The model under review builds one solid part; all positions refer to its coordinate system, in mm. Face numbers are marked on the shaded views. Round coordinates to 2 decimals unless told otherwise and drop trailing zeros. Write each loop counter-clockwise with the first axis right and the second up, starting at its lowest first coordinate (ties: lowest second). Pieces come first, ordered by that corner, then holes. Notation, with made-up numbers: M 85,61 L 126,61 A17 cw 126,91 Z; hole C -19.75,-6 d7. An arc over 180 degrees is marked long. One line per item, written item: value. Start each with the question number.
1) For P1, Ø3, axis at y = 4, z = 5, coming from the +X side; P2, Ø10, axis at x = -10, y = -1, coming from the +Z side; P3, Ø1, axis at y = 5.5, z = 5.5, coming from the +X side, all flat-tipped, find the tip position at first contact; note any pin that passes through.
2) Mouldability with a two-part tool opening along Y and no side actions: class the marked faces 1, 2, 3 and 4 as +Y half, -Y half, draft (parallel to the pull), parting line (faces both ways), or undercut.
3) Wall thickness on probe 1 along Y at (x, z) = (-14.5, 4.75); probe 2 along X at (y, z) = (-3.25, 1.75); probe 3 along X at (y, z) = (5, 3): over which ranges is each line inside the solid? List them lowest first.
4) Take a section at D-D, the plane x = 19. Write out the cut boundary in (y, z), and give its area (3 significant figures).
5) Take a section at B-B, the plane x = 9.5. Write out the cut boundary in (y, z).
6) Take a section at A-A, the plane y = 0. Write out the cut boundary in (x, z), and give its area (3 significant figures).
7) Take a section at C-C, the plane z = 3. Write out the cut boundary in (x, y), and give its area (3 significant figures).
from build123d import *

# Parameters (mm, degrees)
EXTRUDE_1_DEPTH = 7
M16X1_51_D      = 14.5


with BuildPart() as part:
    # Эскиз1 → Бобышка-Вытянуть1 (new body)
    with BuildSketch(Plane.XY):
        with BuildLine():
            Line((14.5, 9), (-14.5, 9))
            ThreePointArc((-14.5, 9), (-23.5, 0), (-14.5, -9))
            Line((-14.5, -9), (14.5, -9))
            ThreePointArc((14.5, -9), (23.5, 0), (14.5, 9))
        make_face()
    extrude(amount=EXTRUDE_1_DEPTH)

    # Отверстие обработанное метчиком M16x1.51 (through all)
    with Locations(Plane(origin=(0, 0, 0), x_dir=(-1, 0, 0), z_dir=(0, 0, -1))):
        with Locations((14.5, 0)):
            m16x1_51 = Hole(M16X1_51_D / 2)

    # Зеркальное отражение1: Отверстие обработанное метчиком M16x1.51 across plane
    add(m16x1_51.mirror(Plane(origin=(0, 0, 0), x_dir=(0, 0, 1), z_dir=(1, 0, 0))), mode=Mode.SUBTRACT)


solid = part.part
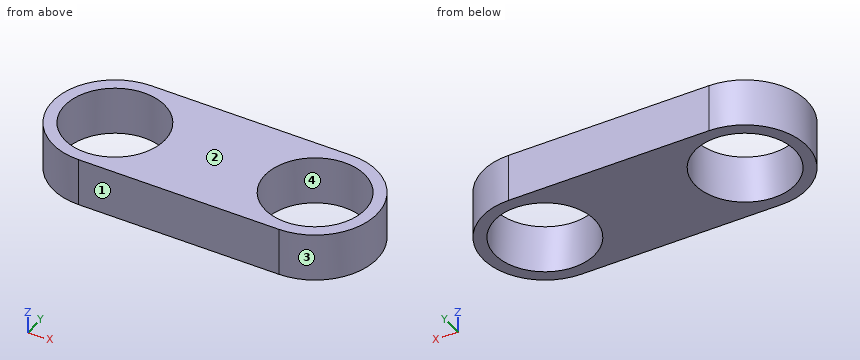
Checked values:
1. P1: stops at x = 23.15
1. P2: stops at z = 7
1. P3: stops at x = 21.98
2. face 1: -Y half
2. face 2: draft
2. face 3: parting line
2. face 4: undercut
3. probe 1: y = -9 to -7.25, 7.25 to 9
3. probe 2: x = -22.89 to -20.98, -8.02 to 8.02, 20.98 to 22.89
3. probe 3: x = -21.98 to -19.75, -9.25 to 9.25, 19.75 to 21.98
4. outline: M -7.79,0 L -5.68,0 L -5.68,7 L -7.79,7 Z; M 5.68,0 L 7.79,0 L 7.79,7 L 5.68,7 Z
4. area: 29.5 mm2
5. outline: M -9,0 L -5.25,0 L -5.25,7 L -9,7 Z; M 5.25,0 L 9,0 L 9,7 L 5.25,7 Z
6. outline: M -23.5,0 L -21.75,0 L -21.75,7 L -23.5,7 Z; M -7.25,0 L 7.25,0 L 7.25,7 L -7.25,7 Z; M 21.75,0 L 23.5,0 L 23.5,7 L 21.75,7 Z
6. area: 126 mm2
7. outline: M -14.5,-9 L 14.5,-9 A9 ccw 14.5,9 L -14.5,9 A9 ccw Z; hole C -14.5,0 d14.5; hole C 14.5,0 d14.5
7. area: 446 mm2
